The drawing under review shows one solid part. Ordinate dimensions are in mm from its lowest x, y, z. A direction names the side the tool comes from. Coordinates: 2 decimals unless noted, no trailing zeros. Write each loop counter-clockwise with the first axis right and the second up, starting at its lowest first coordinate (ties: lowest second). Pieces come first, ordered by that corner, then holes. Notation, with made-up numbers: (0, 42.5) - (7, 42.5) arc R22 ccw to (7, 61.5) - close; hole circle Ø4 at (37.25, 40.5). An arc over 180 degrees is marked (long way). Use a Markdown table: item, result.
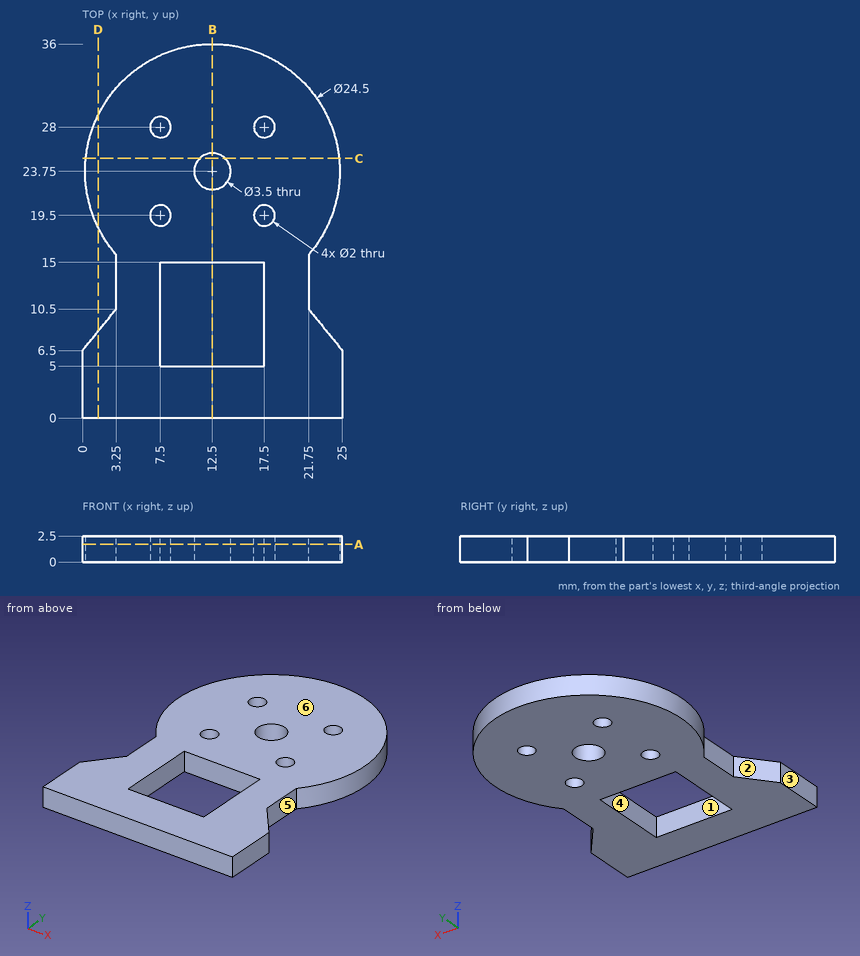
(1) Take a section at B-B on x = 12.5. Write out the cut boundary in (y, z), and give its area (4 significant figures).
Determined:
| item | result |
|---|---|
| outline | (0, 0) - (5, 0) - (5, 2.5) - (0, 2.5) - close; (15, 0) - (22, 0) - (22, 2.5) - (15, 2.5) - close; (25.5, 0) - (36, 0) - (36, 2.5) - (25.5, 2.5) - close |
| area | 56.25 mm2 |
(2) Take a section at C-C on y = 25. Write out the cut boundary in (x, z), and give its area (3 significant figures).
Determined:
| item | result |
|---|---|
| outline | (0.31, 0) - (11.28, 0) - (11.28, 2.5) - (0.31, 2.5) - close; (13.72, 0) - (24.69, 0) - (24.69, 2.5) - (13.72, 2.5) - close |
| area | 54.8 mm2 |
(3) For pin 1 (1.2 mm diameter, centred on y = 9.5, z = 1.5, fed in from +X); pin 2 (1.2 mm diameter, centred on y = 14, z = 1, fed in from -X); pin 3 (1.2 mm diameter, centred on x = 7.5, y = 28, fed in from -Z), all flat-tipped, find the tip position at first contact; note any pin that passes through.
Determined:
| item | result |
|---|---|
| pin 1 | x = 23.05 |
| pin 2 | x = 3.25 |
| pin 3 | through |
(4) Machinability: for the marked faces 1, 2 and 3, which of the approach directions +Z, -Z, +X, -X, +Y, -Y give a long, thin tool a straight path to every point of the face, cutting with its end or side? Answer none if there is none.
Determined:
| item | result |
|---|---|
| face 1 | +Z, -Z |
| face 2 | +Z, -Z, -X |
| face 3 | +Z, -Z, -X, +Y, -Y |
(5) For L1, parallel to Y at x = 12.5, z = 0.8; L2, parallel to X at y = 12, z = 1.5; L3, parallel to X at y = 28.5, z = 1.1, list the stretches that pass through material, from the lowest coordinate up. Write a range as from..to.
Determined:
| item | result |
|---|---|
| L1 | 0..5, 15..22, 25.5..36 |
| L2 | 3.25..7.5, 17.5..21.75 |
| L3 | 1.21..6.63, 8.37..16.63, 18.37..23.79 |
(6) Take a section at D-D on x = 1.5. Write out the cut boundary in (y, z).
Determined:
| item | result |
|---|---|
| outline | (0, 0) - (8.35, 0) - (8.35, 2.5) - (0, 2.5) - close; (18.36, 0) - (29.14, 0) - (29.14, 2.5) - (18.36, 2.5) - close |
(7) Draft analysis for pull direction X (two halves, no side actions). For the marked faces 4, 5 and 6, state which applies: +X half, -X half, draft (parallel to the pull), parting line (faces both ways), or undercut.
Determined:
| item | result |
|---|---|
| face 4 | undercut |
| face 5 | +X half |
| face 6 | draft |
(8) Take a section at A-A on z = 1.7. Write out the cut boundary in (x, y), and give its area (3 significant figures).
Determined:
| item | result |
|---|---|
| outline | (0, 0) - (25, 0) - (25, 6.5) - (21.75, 10.5) - (21.75, 15.72) arc R12.25 ccw (long way) to (3.25, 15.72) - (3.25, 10.5) - (0, 6.5) - close; hole circle Ø2 at (7.5, 19.5); hole circle Ø2 at (7.5, 28); hole (7.5, 5) - (17.5, 5) - (17.5, 15) - (7.5, 15) - close; hole circle Ø3.5 at (12.5, 23.75); hole circle Ø2 at (17.5, 19.5); hole circle Ø2 at (17.5, 28) |
| area | 641 mm2 |
